```python
from build123d import *

# Parameters (mm, degrees)
SKETCH3_R          = 7
CUT_EXTRUDE1_DEPTH = 39.897300678
CHAMFER1_SIZE      = 1


with BuildPart() as part:
    # Sketch1 → Revolve1 (revolve)
    with BuildSketch(Plane.XY, mode=Mode.PRIVATE) as revolve1_sk:
        Polygon((0, 0), (0, -10), (-25, -10), (-25, -12), (-35, -12), (-35, 0), align=None)
    revolve(revolve1_sk.sketch.rotate(Axis((0, 0, 0), (-1, 0, 0)), 180), axis=Axis((0, 0, 0), (-1, 0, 0)))

    # Sketch3 → Cut-Extrude1 (cut, through all)
    with BuildSketch(Plane(origin=(0, 0, 0), x_dir=(0, 0, -1), z_dir=(1, 0, 0))):
        with Locations(Location((0, 0, 0), (0, 0, 90))):
            Circle(SKETCH3_R)
    extrude(amount=-CUT_EXTRUDE1_DEPTH, mode=Mode.SUBTRACT)

    # Chamfer1
    chamfer1_edges = [part.edges().sort_by_distance(p)[0] for p in [
        (-35, -12, 0),
        (0, -10, 0),
    ]]
    chamfer(chamfer1_edges, length=CHAMFER1_SIZE)


solid = part.part
```
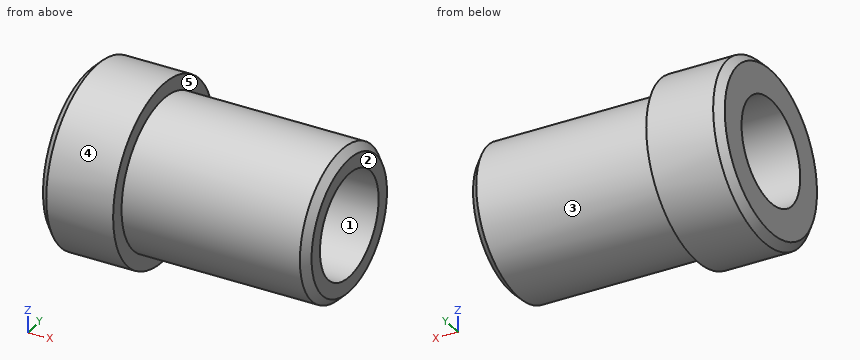
The model under review builds one solid part; all positions refer to its coordinate system, in mm. Face numbers are marked on the shaded views. A direction names the side the tool comes from. Give positions to 0.01 mm unless a question says otherwise; leave off trailing zeros. Write each loop counter-clockwise with the first axis right and the second up, starting at its lowest first coordinate (ties: lowest second). Pieces come first, ordered by that corner, then holes. Notation, with made-up numbers: (9, -29.75) - (62, -29.75) arc R22 ccw to (62, -22.75) - close; hole circle Ø7 at (-22, 37.5). An arc over 180 degrees is marked (long way). Answer in a Markdown table with one row per item. Add a question column.
1. Wall thickness on line 1 along Z through (x, y) = (-19, 0); line 2 along Z through (x, y) = (-9, -5.5): over which ranges is each line inside the solid? List them lowest first. Write a range as [from, to].
2. Insertion check: P1, Ø1, axis at x = -12, y = -1.5, coming from the -Z side; P2, Ø5, axis at x = -7, z = 7.5, coming from the -Y side; P3, Ø6, axis at x = -16, z = 0, coming from the -Y side; P4, Ø5, axis at y = 2.5, z = 1.5, coming from the +X side. Each pin has a flat end and moves straight along its axis. Give the tip position at first contact, or say it passes through.
3. Tool access review of the marked faces 4 and 5: name each direction out of +Z, -Z, +X, -X, +Y, -Y from which nothing blocks a thin tool from reaching the whole face with its end or side.
4. Draft analysis for pull direction Z (two halves, no side actions). For the marked faces 1, 2 and 3, state which applies: +Z half, -Z half, draft (parallel to the pull), parting line (faces both ways), or undercut.
5. We need section A-A on z = 0. Write out the cut boundary in (x, y).
6. We need section C-C on x = -12. Write out the cut boundary in (y, z).
Ans:
| question | item | result |
|---|---|---|
| 1 | line 1 | z = [-10, -7], [7, 10] |
| 1 | line 2 | z = [-8.35, -4.33], [4.33, 8.35] |
| 2 | P1 | stops at z = -9.95 |
| 2 | P2 | stops at y = -8.66 |
| 2 | P3 | stops at y = -10 |
| 2 | P4 | passes through |
| 3 | face 4 | +X, -X |
| 3 | face 5 | +X |
| 4 | face 1 | undercut |
| 4 | face 2 | draft |
| 4 | face 3 | parting line |
| 5 | outline | (-35, -11) - (-34, -12) - (-25, -12) - (-25, -10) - (-1, -10) - (0, -9) - (0, -7) - (-35, -7) - close; (-35, 7) - (0, 7) - (0, 9) - (-1, 10) - (-25, 10) - (-25, 12) - (-34, 12) - (-35, 11) - close |
| 6 | outline | circle Ø20 at (0, 0); hole circle Ø14 at (0, 0) |
